Verification items for the finished model (mm, model axes). A direction names the side the tool comes from. Coordinates: 2 decimals unless noted, no trailing zeros. Write each loop counter-clockwise with the first axis right and the second up, starting at its lowest first coordinate (ties: lowest second). Pieces come first, ordered by that corner, then holes. Notation, with made-up numbers: (-31.5, -12.5) - (7.5, -12.5) arc R14 cw to (7.5, 7.5) - close; hole circle Ø2 at (20.5, 41). An arc over 180 degrees is marked (long way). Answer as CSV lines item,"result". Start each with the question number.
```python
from build123d import *

# Parameters (mm, degrees)
SKETCH2_W               = 48.66
SKETCH2_H               = 48.36
BOSS_EXTRUDE1_DEPTH     = 43.2689
SKETCH3_W               = 37.992
SKETCH3_H               = 8.128
CUT_EXTRUDE1_DEPTH      = 38.1889
SKETCH4_W               = 38.5064
SKETCH4_H               = 38.608
CUT_EXTRUDE2_DEPTH      = 33.1089
SKETCH6_R               = 2.794
CUT_EXTRUDE3_DEPTH      = 78.486
CUT_EXTRUDE3_DEPTH_BACK = 23.622
SKETCH7_W               = 30.48
SKETCH7_H               = 6.35
BOSS_EXTRUDE2_DEPTH     = 7.62
SKETCH9_W               = 6.35
SKETCH9_H               = 50.8
BOSS_EXTRUDE3_DEPTH     = 30.48
SKETCH11_W              = 101.6
SKETCH11_H              = 38.1
BOSS_EXTRUDE4_DEPTH     = 13.97
SKETCH14_R              = 1.778
CUT_EXTRUDE4_DEPTH      = 13.97
FILLET1_R               = 2.54
SKETCH15_W              = 6.604
SKETCH15_H              = 6.604
CUT_EXTRUDE5_DEPTH      = 3.302


with BuildPart() as part:
    # Sketch2 → Boss-Extrude1 (new body)
    with BuildSketch(Plane.XY):
        with Locations((19.25, 19.1)):
            Rectangle(SKETCH2_W, SKETCH2_H)
    extrude(amount=BOSS_EXTRUDE1_DEPTH)

    # Sketch3 → Cut-Extrude1 (cut)
    with BuildSketch(Plane(origin=(0, 0, 0), x_dir=(-1, 0, 0), z_dir=(0, 0, -1))):
        with Locations((-18.996, 4.064)):
            Rectangle(SKETCH3_W, SKETCH3_H)
    extrude(amount=-CUT_EXTRUDE1_DEPTH, mode=Mode.SUBTRACT)

    # Sketch4 → Cut-Extrude2 (cut)
    with BuildSketch(Plane.XY.offset(43.2689)):
        with Locations((19.2468, 19.304)):
            Rectangle(SKETCH4_W, SKETCH4_H)
    extrude(amount=-CUT_EXTRUDE2_DEPTH, mode=Mode.SUBTRACT)

    # Sketch6 → Cut-Extrude3 (cut, two sides)
    with BuildSketch(Plane.ZY.offset(-38.5)) as cut_extrude3_sk:
        with Locations((17.714319607, 19.508)):
            Circle(SKETCH6_R)
    extrude(amount=CUT_EXTRUDE3_DEPTH, mode=Mode.SUBTRACT)
    extrude(cut_extrude3_sk.sketch, amount=-CUT_EXTRUDE3_DEPTH_BACK, mode=Mode.SUBTRACT)

    # Sketch7 → Boss-Extrude2 (add)
    with BuildSketch(Plane(origin=(43.58, 0, 0), x_dir=(0, 0, -1), z_dir=(1, 0, 0))):
        with Locations((-21.63445, 1.905)):
            Rectangle(SKETCH7_W, SKETCH7_H)
    boss_extrude2 = extrude(amount=BOSS_EXTRUDE2_DEPTH)

    # Sketch9 → Boss-Extrude3 (add)
    with BuildSketch(Plane.XY.offset(36.87445)):
        with Locations((48.025, -26.67)):
            Rectangle(SKETCH9_W, SKETCH9_H)
    boss_extrude3 = extrude(amount=-BOSS_EXTRUDE3_DEPTH)

    # Mirror1: Boss-Extrude2, Boss-Extrude3 across plane
    add(boss_extrude2.mirror(Plane(origin=(19.25, 0, 0), x_dir=(0, 0, 1), z_dir=(1, 0, 0))))
    add(boss_extrude3.mirror(Plane(origin=(19.25, 0, 0), x_dir=(0, 0, 1), z_dir=(1, 0, 0))))

    # Sketch11 → Boss-Extrude4 (add)
    with BuildSketch(Plane.XZ.offset(52.07)):
        with Locations((19.25, 21.63445)):
            Rectangle(SKETCH11_W, SKETCH11_H)
    extrude(amount=BOSS_EXTRUDE4_DEPTH)

    # Sketch14 → Cut-Extrude4 (cut)
    with BuildSketch(Plane.XZ.offset(66.04)):
        with Locations((57.376985722, 21.63445)):
            Circle(SKETCH14_R)
        with Locations((-18.876985722, 21.63445)):
            Circle(SKETCH14_R)
    extrude(amount=-CUT_EXTRUDE4_DEPTH, mode=Mode.SUBTRACT)

    # Fillet1
    fillet1_edges = [part.edges().sort_by_distance(p)[0] for p in [
        (-12.7, -52.07, 21.63445),
        (51.2, -52.07, 21.63445),
    ]]
    fillet(fillet1_edges, radius=FILLET1_R)

    # Sketch15 → Cut-Extrude5 (cut)
    with BuildSketch(Plane(origin=(0, 43.28, 0), x_dir=(1, 0, 0), z_dir=(0, 1, 0))):
        with Locations((19.25, -21.63445)):
            Rectangle(SKETCH15_W, SKETCH15_H)
    extrude(amount=-CUT_EXTRUDE5_DEPTH, mode=Mode.SUBTRACT)


solid = part.part
```
1. Access from +Z, -Z, +X, -X, +Y, -Y to the whole of each face (thin tool, end or side, straight path). Record for faces 1 (the face through (47, -23, 36.874)), 2 (the face through (44.85, -27, 22)), 3 (the face through (19, 24, 10.16)).
2. Cross-section at A-A (y = -44). Record the cut outline in (x, z), and give its area (3 significant figures).
3. Cross-section at D-D (x = 24). Record the cut outline in (y, z), and give its area (3 significant figures).
4. Scan lines: line 1 along Y through (x, z) = (22, 19.5); line 2 along Y through (x, z) = (23.5, 37.5); line 3 along X through (y, z) = (4, 5). Record each from-to range of solid material in increasing order. Write a range as from..to.
5. Cross-section at C-C (z = 35.5). Record the cut outline in (x, y).
6. Cross-section at B-B (x = -9.5). Record the cut outline in (y, z), and give its area (3 significant figures).
7. Draft check along X on faces 4 (the face through (-13.464, -51.346, 21.421)), 5 (the face through (19, 8.128, 5)), 6 (the face through (19, -59, 2.584)). Enter one of: pulls with the +X half, pulls with the -X half, needs draft (parallel to the pull), parting line crosses it, or undercut.
8. Depth check by flat-ended pin: P1, Ø4, axis at y = 3.5, z = 4.5, coming from the -X side; P2, Ø24.5, axis at y = -25.5, z = 17, coming from the +X side; P3, Ø19.5, axis at x = 11.5, y = 11, coming from the +Z side. Enter the tip coordinate at first touch or a pass-through.
Completed:
1,face 1,"+Z, +X, +Y"
1,face 2,"+Z, -Z"
1,face 3,"+Z"
2,outline,"(-12.7, 6.39) - (-6.35, 6.39) - (-6.35, 36.87) - (-12.7, 36.87) - close; (44.85, 6.39) - (51.2, 6.39) - (51.2, 36.87) - (44.85, 36.87) - close"
2,area,"387 mm2"
3,outline,"(-66.04, 2.58) - (-52.07, 2.58) - (-52.07, 40.68) - (-66.04, 40.68) - close; (-5.08, 0) - (0, 0) - (0, 43.27) - (-5.08, 43.27) - close; (8.13, 0) - (43.28, 0) - (43.28, 43.27) - (38.61, 43.27) - (38.61, 10.16) - (8.13, 10.16) - close"
3,area,"1,260 mm2"
4,line 1,"y = -66.04..-52.07, -5.08..0, 38.61..39.98"
4,line 2,"y = -66.04..-52.07, -5.08..0, 38.61..43.28"
4,line 3,"x = -5.08..0, 37.99..43.58"
5,outline,"(-31.55, -66.04) - (70.05, -66.04) - (70.05, -52.07) - (53.74, -52.07) arc R2.54 cw to (51.2, -49.53) - (51.2, 5.08) - (43.58, 5.08) - (43.58, 43.28) - (-5.08, 43.28) - (-5.08, 5.08) - (-12.7, 5.08) - (-12.7, -49.53) arc R2.54 cw to (-15.24, -52.07) - (-31.55, -52.07) - close; hole (-6.35, -52.07) - (44.85, -52.07) - (44.85, -1.27) - (43.58, -1.27) - (43.58, -5.08) - (-5.08, -5.08) - (-5.08, -1.27) - (-6.35, -1.27) - close; hole (-0.01, 0) - (38.5, 0) - (38.5, 38.61) - (-0.01, 38.61) - close"
6,outline,"(-66.04, 2.58) - (-52.07, 2.58) - (-52.07, 6.39) - (5.08, 6.39) - (5.08, 36.87) - (-52.07, 36.87) - (-52.07, 40.68) - (-66.04, 40.68) - close"
6,area,"2,270 mm2"
7,face 4,"pulls with the -X half"
7,face 5,"undercut"
7,face 6,"needs draft"
8,P1,"stops at x = -12.7"
8,P2,"stops at x = 51.2"
8,P3,"stops at z = 10.16"
